```python
from build123d import *

# Parameters (mm, degrees)
SKETCH016_W     = 40
SKETCH016_H     = 40
PAD005_DEPTH    = 8
FILLET003_R     = 5
SKETCH017_W     = 22.5
SKETCH017_H     = 12.3
POCKET011_DEPTH = 4
SKETCH018_R     = 3
POCKET012_DEPTH = 5
SKETCH019_W     = 7
SKETCH019_H     = 3
POCKET013_DEPTH = 8


with BuildPart() as part:
    # Sketch016 → Pad005 (new body)
    with BuildSketch(Plane.XY):
        Rectangle(SKETCH016_W, SKETCH016_H)
    extrude(amount=PAD005_DEPTH)

    # Fillet003
    fillet003_edges = [part.edges().sort_by_distance(p)[0] for p in [
        (-20, -20, 4),
        (20, -20, 4),
        (20, 20, 4),
        (-20, 20, 4),
    ]]
    fillet(fillet003_edges, radius=FILLET003_R)

    # Sketch017 (on Face2 of Fillet003) → Pocket011 (cut)
    with BuildSketch(Plane(origin=(0, 0, 0), x_dir=(1, 0, 0), z_dir=(0, 0, -1))):
        with Locations((5.05, 0)):
            Rectangle(SKETCH017_W, SKETCH017_H)
    extrude(amount=-POCKET011_DEPTH, mode=Mode.SUBTRACT)

    # Sketch018 (on Face5 of Pocket011) → Pocket012 (cut)
    with BuildSketch(Plane.XY.offset(8)):
        Circle(SKETCH018_R)
    extrude(amount=-POCKET012_DEPTH, mode=Mode.SUBTRACT)

    # Sketch019 (on Face2 of Pocket012) → Pocket013 (cut)
    with BuildSketch(Plane(origin=(0, 0, 0), x_dir=(1, 0, 0), z_dir=(0, 0, -1))):
        with Locations((0, -13.263275)):
            Rectangle(SKETCH019_W, SKETCH019_H)
    extrude(amount=-POCKET013_DEPTH, mode=Mode.SUBTRACT)


with BuildPart() as part_1:
    # Body002 placement: moved
    add(part.part.moved(Location((0, 0, 38))))


solid = part_1.part
```
Verification items for the finished model (mm, model axes). A direction names the side the tool comes from. Round coordinates to 2 decimals unless told otherwise and drop trailing zeros. Write each loop counter-clockwise with the first axis right and the second up, starting at its lowest first coordinate (ties: lowest second). Pieces come first, ordered by that corner, then holes. Notation, with made-up numbers: (70, 47) -> (119, 47) arc R16 cw to (119, 59) -> close; hole circle Ø10 at (25.5, -28). An arc over 180 degrees is marked (long way). Write each question's results on one line, items separated by ' | '. Start each with the question number.
1. Set-up check for faces 1 (the flat face through (5, -6.15, 40)), 2 (the flat face through (3.5, 13, 42)), 3 (the cylindrical face through (-19, -18, 42)): record each of +Z, -Z, +X, -X, +Y, -Y from which the full face is reachable in a straight line by a thin tool's end or side.
2. Cross-section at D-D (x = -5). Enter the section's corners in (y, z).
3. Draft check along Y on faces 4 (the cylindrical face through (19, 18, 42)), 5 (the cylindrical face through (18, -19, 42)), 6 (the flat face through (0, 11.763, 42)), 7 (the flat face through (-6.2, 0, 40)). Enter one of: +Y half, -Y half, draft (parallel to the pull), parting line (faces both ways), or undercut.
4. Depth check by flat-ended pin: P1, Ø6, axis at x = 3.5, y = -3, coming from the -Z side. Enter the tip coordinate at first touch or a pass-through.
5. Cross-section at A-A (y = 0). Enter the section's corners in (x, z), then the cut area to 3 significant figures.
6. Cross-section at B-B (z = 39.5). Enter the section's corners in (x, y).
7. Cross-section at C-C (x = 0). Enter the section's corners in (y, z).
8. Material ranges on probe 1 along Y at (x, z) = (0, 44.5); probe 2 along X at (y, z) = (12.5, 43); probe 3 along Z at (x, y) = (-1, 3.5), recorded low to high. Write a range as from..to.
Solutions:
1) face 1: -Z | face 2: +Z, -Z | face 3: +Z, -Z, -X, -Y
2) outline: (-20, 38) -> (-6.15, 38) -> (-6.15, 42) -> (6.15, 42) -> (6.15, 38) -> (20, 38) -> (20, 46) -> (-20, 46) -> close
3) face 4: +Y half | face 5: -Y half | face 6: undercut | face 7: undercut
4) P1: stops at z = 42
5) outline: (-20, 38) -> (-6.2, 38) -> (-6.2, 42) -> (-3, 42) -> (-3, 46) -> (-20, 46) -> close; (3, 42) -> (16.3, 42) -> (16.3, 38) -> (20, 38) -> (20, 46) -> (3, 46) -> close | area: 206 mm2
6) outline: (-20, -15) arc R5 ccw to (-15, -20) -> (15, -20) arc R5 ccw to (20, -15) -> (20, 15) arc R5 ccw to (15, 20) -> (-15, 20) arc R5 ccw to (-20, 15) -> close; hole (-6.2, -6.15) -> (16.3, -6.15) -> (16.3, 6.15) -> (-6.2, 6.15) -> close; hole (-3.5, 11.76) -> (3.5, 11.76) -> (3.5, 14.76) -> (-3.5, 14.76) -> close
7) outline: (-20, 38) -> (-6.15, 38) -> (-6.15, 42) -> (-3, 42) -> (-3, 46) -> (-20, 46) -> close; (3, 42) -> (6.15, 42) -> (6.15, 38) -> (11.76, 38) -> (11.76, 46) -> (3, 46) -> close; (14.76, 38) -> (20, 38) -> (20, 46) -> (14.76, 46) -> close
8) probe 1: y = -20..-3, 3..11.76, 14.76..20 | probe 2: x = -20..-3.5, 3.5..20 | probe 3: z = 42..46
